CAD build for the part. Positions are in the model's coordinates, mm. A direction names the side the tool comes from. Coordinates: 2 decimals unless noted, no trailing zeros. Order: outer loops, then holes, each group sorted by start corner. A loop starts at its lowest first (then second) coordinate and runs counter-clockwise, first axis right, second up. Notation, with made-up numbers: (88, 16.5) - (102, 16.5) arc R10 ccw to (102, 24.5) - close; hole circle Ø3 at (-10, 66). An arc over 180 degrees is marked (long way). Use one line per item in the form item = value.
```python
from build123d import *

# Parameters (mm, degrees)
BOSS_EXTRUDE1_DEPTH = 12.7
SKETCH2_R           = 1.7526
CUT_EXTRUDE3_DEPTH  = 4.175
SKETCH3_R           = 1.7526
CUT_EXTRUDE4_DEPTH  = 4.436950898


with BuildPart() as part:
    # Sketch1 → Boss-Extrude1 (new body)
    with BuildSketch(Plane.XY):
        Polygon((-5.5, -6.5), (-19.05, -6.5), (-19.05, -3.325), (-8.675, -3.325), (-8.675, 10.645), (8.675, 10.645), (8.675, -3.063049102), (19.05, -3.063049102), (19.05, -6.5), (5.5, -6.5), (5.5, 6.5), (-5.5, 6.5), align=None)
    extrude(amount=BOSS_EXTRUDE1_DEPTH)

    # Sketch2 → Cut-Extrude3 (cut, through all)
    with BuildSketch(Plane(origin=(0, -3.325, 0), x_dir=(1, 0, 0), z_dir=(0, 1, 0))):
        with Locations((-13.97, -6.35)):
            Circle(SKETCH2_R)
    extrude(amount=-CUT_EXTRUDE3_DEPTH, mode=Mode.SUBTRACT)

    # Sketch3 → Cut-Extrude4 (cut, through all)
    with BuildSketch(Plane(origin=(0, -3.063049102, 0), x_dir=(1, 0, 0), z_dir=(0, 1, 0))):
        with Locations((13.97, -6.35)):
            Circle(SKETCH3_R)
    extrude(amount=-CUT_EXTRUDE4_DEPTH, mode=Mode.SUBTRACT)


solid = part.part
```
Item 1: Drill centre lines: line 1 (X direction, y = -5.6, z = 6.35); line 2 (X direction, y = 6, z = 5.5) (3 decimals); line 3 (Z direction, x = -13.97, y = -4.1). Where is each one in solid material? Low to high. Write a range as [from, to].
Derived:
line_1 = [-19.05, -15.72], [-12.22, -5.5], [5.5, 12.22], [15.72, 19.05]
line_2 = [-8.675, -5.5], [5.5, 8.675]
line_3 = [0, 4.6], [8.1, 12.7]
Item 2: Cut at C-C, the plane z = 10. Write the cut outline in (x, y) (3 decimals), plus the area to 3 significant figures.
Derived:
outline = (-19.05, -6.5) - (-5.5, -6.5) - (-5.5, 6.5) - (5.5, 6.5) - (5.5, -6.5) - (19.05, -6.5) - (19.05, -3.063) - (8.675, -3.063) - (8.675, 10.645) - (-8.675, 10.645) - (-8.675, -3.325) - (-19.05, -3.325) - close
area = 223 mm²
Item 3: Cut at D-D, the plane x = -2. Write the cut outline in (y, z) (3 decimals).
Derived:
outline = (6.5, 0) - (10.645, 0) - (10.645, 12.7) - (6.5, 12.7) - close
Item 4: Cut at B-B, the plane y = 3. Write the cut outline in (x, z) (3 decimals), plus the area to 3 significant figures.
Derived:
outline = (-8.675, 0) - (-5.5, 0) - (-5.5, 12.7) - (-8.675, 12.7) - close; (5.5, 0) - (8.675, 0) - (8.675, 12.7) - (5.5, 12.7) - close
area = 80.6 mm²
Item 5: Cut at A-A, the plane x = -13.97. Write the cut outline in (y, z) (3 decimals), plus the area to 3 significant figures.
Derived:
outline = (-6.5, 0) - (-3.325, 0) - (-3.325, 4.597) - (-6.5, 4.597) - close; (-6.5, 8.103) - (-3.325, 8.103) - (-3.325, 12.7) - (-6.5, 12.7) - close
area = 29.2 mm²
Item 6: Drop flat-ended pins along their axis: pin 1 (6.5 mm diameter, centred on y = 0.5, z = 9.5, fed in from +X) (3 decimals); pin 2 (3 mm diameter, centred on x = -15.5, z = 3.5, fed in from +Y) (3 decimals); pin 3 (4.5 mm diameter, centred on x = -13.97, z = 6.35, fed in from -Y); pin 4 (3.5 mm diameter, centred on x = -2, z = 7, fed in from -Y). Give the stop position or say it passes through.
Derived:
pin_1 = 8.675
pin_2 = -3.325
pin_3 = -6.5
pin_4 = 6.5
Item 7: 3-axis set-ups, long thin cutter, end or side, ignore diameter. For faces 5 (the face through (0, 6.5, 6)), 6 (the face through (-12.8, -3.325, 4.8)), 7 (the face through (12.6, -3.063, 4.8)): which of +Z, -Z, +X, -X, +Y, -Y reach the whole face in a straight line?
Derived:
face_5 = +Z, -Z, -Y
face_6 = +Z, -Z, -X, +Y
face_7 = +Z, -Z, +X, +Y
Item 8: Two-plate mould, pull along X, no slides. Class faces 1 (the face through (14.91, -4.76, 4.87)), 2 (the face through (-5.5, 0, 6)), 3 (the face through (-12, -6.5, 6)), 4 (the face through (-8.675, 4, 6)): +X half, -X half, draft (parallel to the pull), parting line (faces both ways), or undercut.
Derived:
face_1 = undercut
face_2 = undercut
face_3 = draft
face_4 = -X half
